Autodesk Inventor part; units mm, degrees
ref_plane "YZ Plane" through (0, 0, 0) normal (1, 0, 0) x (0, 1, 0)
ref_plane "XZ Plane" through (0, 0, 0) normal (0, 1, 0) x (-1, 0, 0)
ref_plane "XY Plane" through (0, 0, 0) normal (0, 0, 1) x (1, 0, 0)
sketch "Sketch1" plane through (0, 0, 0) normal (0, 0, 1) x (1, 0, 0)
  line L0 (-6.5, 1) -> (6.5, 1)
  line L1 (6.5, 1) -> (6.5, -1)
  line L2 (6.5, -1) -> (-6.5, -1)
  line L3 (-6.5, -1) -> (-6.5, 1)
  circle A0 centre (-5.5, 0) radius 0.25
  circle A1 centre (5.5, 0) radius 0.5
  point P0 (0, 0)
  point P1 (0, 1)
  point P2 (-6.5, 0)
  dimension "d0" = 2
  dimension "d1" = 0.5
  dimension "d2" = 1
  dimension "d7" = 13
  dimension "d8" = 1
  dimension "d12" = 1
extrude "Extrusion1" add sketch "Sketch1" along normal mid plane 0.5
fillet "Fillet1" radius 1 4 edges at (6.5, 1, 0) (6.5, -1, 0) (-6.5, 1, 0) (-6.5, -1, 0)
sketch "Sketch3" plane through (0, 0, 0.25) normal (0, 0, 1) x (1, 0, 0)
  circle A0 centre (5.5, 0) radius 0.5
  circle A1 centre (5.5, 0) radius 0.65
  point P0 (0, 0)
  dimension "d13" = 1.3
extrude "Extrusion2" add sketch "Sketch3" along normal blind 0.15
chamfer "Chamfer1" distance 0.15 angle 45 1 edges at (4.85, 0, 0.4)
fillet "Fillet2" radius 0.25 8 edges at (-6.2073, 0.7073, -0.25) (0, 1, -0.25) (6.2073, 0.7073, -0.25) (0, -1, -0.25) (6.2073, 0.7073, 0.25) (0, 1, 0.25) (-6.2073, 0.7073, 0.25) (0, -1, 0.25)
sketch "Sketch4" plane through (0, 0, -0.25) normal (0, 0, -1) x (-1, 0, 0)
  circle A0 centre (5.5, 0) radius 0.25
  circle A1 centre (5.5, 0) radius 0.375
  point P0 (0, 0)
  dimension "d20" = 0.75
extrude "Extrusion3" cut sketch "Sketch4" against normal blind 0.15
chamfer "Chamfer3" distance 0.1 angle 45 1 edges at (-5.125, 0, -0.25)
properties part number "Link_2"
Could you check a few things on this model? Use its own coordinates, in mm. Coordinates: 2 decimals unless noted, no trailing zeros.
Q1. Please list where these lines run through material, in increasing order: L1, parallel to Y at x = 5.5, z = 0; L2, parallel to Y at x = -5.5, z = 0.05; L3, parallel to Z at x = 3.75, y = 0.45.
Q2. Thinking about a two-plate mould opening in Y: for faces 1 (the cylindrical face through (5, 0, 0)), 2 (the flat face through (0, 0, 0.25)), which applies, released by +Y, released by -Y, zero draft, split by the parting line, or undercut?
Q3. Will this pin go through, and if not, where does the flat tip stop? pin 1 (0.8 mm diameter, centred on x = -2, y = 0, fed in from +Z).
Answer:
1. L1: y = -1 to -0.5, 0.5 to 1
1. L2: y = -1 to -0.25, 0.25 to 1
1. L3: z = -0.25 to 0.25
2. face 1: undercut
2. face 2: zero draft
3. pin 1: stops at z = 0.25
